Can you work these out from the model? Positions are in its coordinate system, mm. Round coordinates to 2 decimals unless told otherwise and drop trailing zeros. Order: outer loops, then holes, each group sorted by start corner. A loop starts at its lowest first (then second) coordinate and runs counter-clockwise, first axis right, second up.
from build123d import *

# Parameters (mm, degrees)
F0_W     = 34
F0_H     = 26
F1_DEPTH = 13
F3_DEPTH = 25


with BuildPart() as f1:
    # F0 (on Top) → F1 (new body)
    with BuildSketch(Plane.XY):
        with Locations((17, 13)):
            Rectangle(F0_W, F0_H)
    extrude(amount=F1_DEPTH)

    # F2 (on face) → F3 (cut)
    with BuildSketch(Plane.XY.offset(13)):
        with BuildLine():
            Line((5.1, 21.7), (3.4, 21.7))
            ThreePointArc((3.4, 21.7), (5.1, 20), (6.8, 21.7))
            ThreePointArc((6.8, 21.7), (6.302082, 22.902082), (5.1, 23.4))
            Line((5.1, 23.4), (5.1, 21.7))
        make_face()
        with BuildLine():
            ThreePointArc((28.9, 23.35), (27.733274, 20.533274), (30.55, 21.7))
            Line((30.55, 21.7), (28.9, 21.7))
            Line((28.9, 21.7), (28.9, 23.35))
        make_face()
        with BuildLine():
            ThreePointArc((30.6, 4.3), (27.697918, 5.502082), (28.9, 2.6))
            Line((28.9, 2.6), (28.9, 4.3))
            Line((28.9, 4.3), (30.6, 4.3))
        make_face()
        with BuildLine():
            Line((5.1, 4.3), (5.1, 2.6))
            ThreePointArc((5.1, 2.6), (6.302082, 3.097918), (6.8, 4.3))
            ThreePointArc((6.8, 4.3), (5.1, 6), (3.4, 4.3))
            Line((3.4, 4.3), (5.1, 4.3))
        make_face()
        with BuildLine():
            ThreePointArc((3.4, 4.3), (3.897918, 3.097918), (5.1, 2.6))
            Line((5.1, 2.6), (5.1, 4.3))
            Line((5.1, 4.3), (3.4, 4.3))
        make_face()
        with BuildLine():
            Line((28.9, 4.3), (28.9, 2.6))
            ThreePointArc((28.9, 2.6), (30.102082, 3.097918), (30.6, 4.3))
            Line((30.6, 4.3), (28.9, 4.3))
        make_face()
        with BuildLine():
            Line((28.9, 21.7), (30.55, 21.7))
            ThreePointArc((30.55, 21.7), (30.066726, 22.866726), (28.9, 23.35))
            Line((28.9, 23.35), (28.9, 21.7))
        make_face()
        with BuildLine():
            ThreePointArc((5.1, 23.4), (3.897918, 22.902082), (3.4, 21.7))
            Line((3.4, 21.7), (5.1, 21.7))
            Line((5.1, 21.7), (5.1, 23.4))
        make_face()
    extrude(amount=-F3_DEPTH, mode=Mode.SUBTRACT)


solid = f1.part
(1) Please list where these lines run through material, in increasing order: probe 1 along Y at (x, z) = (28.9, 9.75); probe 2 along X at (y, z) = (21.7, 6.25); probe 3 along X at (y, z) = (5, 0.5).
(2) I want a section at C-C, the plane y = 21. List the corners of the cut face in (x, z) for me.
(3) I want a section at B-B, the plane x = 28.5. List the corners of the cut face in (y, z) for me, plus the area to 3 significant figures.
(4) I want a section at A-A, the plane z = 11.75. List the corners of the cut face in (x, y) for me, plus the area to 3 significant figures.
Ans:
1. probe 1: y = 0 to 2.6, 6 to 20.05, 23.35 to 26
1. probe 2: x = 0 to 3.4, 6.8 to 27.25, 30.55 to 34
1. probe 3: x = 0 to 3.55, 6.65 to 27.35, 30.45 to 34
2. outline: (0, 0) - (3.55, 0) - (3.55, 13) - (0, 13) - close; (6.65, 0) - (27.41, 0) - (27.41, 13) - (6.65, 13) - close; (30.39, 0) - (34, 0) - (34, 13) - (30.39, 13) - close
3. outline: (0, 0) - (2.65, 0) - (2.65, 13) - (0, 13) - close; (5.95, 0) - (20.1, 0) - (20.1, 13) - (5.95, 13) - close; (23.3, 0) - (26, 0) - (26, 13) - (23.3, 13) - close
3. area: 253 mm2
4. outline: (0, 0) - (34, 0) - (34, 26) - (0, 26) - close; hole (3.4, 4.3) arc R1.7 ccw to (5.1, 2.6) arc R1.7 ccw to (6.8, 4.3) arc R1.7 ccw to start; hole (3.4, 21.7) arc R1.7 ccw to (6.8, 21.7) arc R1.7 ccw to (5.1, 23.4) arc R1.7 ccw to start; hole circle Ø3.3 at (28.9, 21.7); hole (28.9, 2.6) arc R1.7 ccw to (30.6, 4.3) arc R1.7 ccw (long way) to start
4. area: 848 mm2
